Study the drawing (mm; zero at the part's minimum x, y, z) and answer. A direction names the side the tool comes from. Give positions to 0.01 mm unless a question says otherwise; leave off trailing zeros. Write each loop counter-clockwise with the first axis right and the second up, starting at its lowest first coordinate (ties: lowest second). Pieces come first, ordered by that corner, then holes.
1) Given pin 1 Ø1.5 at (y, z) = (9, 5) entering from -X; pin 2 Ø12 at (x, z) = (3, 5.5) entering from +Y; pin 3 Ø2 at (x, y) = (4.5, 14.5) entering from +Z, each flat-ended and moving along its own axis, determine where each tip first touches the part or whether it passes through.
2) Find section C-C (z = 16.5). Determine the outline of the cut face in (x, y).
3) Find section D-D (z = 6.5). Determine the outline of the cut face in (x, y).
4) A tool of negligible diameter and unlimited length cuts with its end or side. For the marked faces 1 and 2, from which of +Z, -Z, +X, -X, +Y, -Y can it reach the whole face along a straight path? Write none if from no direction.
5) Find section A-A (x = 12.5). Determine the outline of the cut face in (y, z).
6) Straight lines are drawn through the part: probe 1 along Z at (x, y) = (22.5, 14); probe 2 along X at (y, z) = (12.25, 5); probe 3 along Y at (x, z) = (14, 1.75). For each, find the intervals that lie inside material, in ascending order.
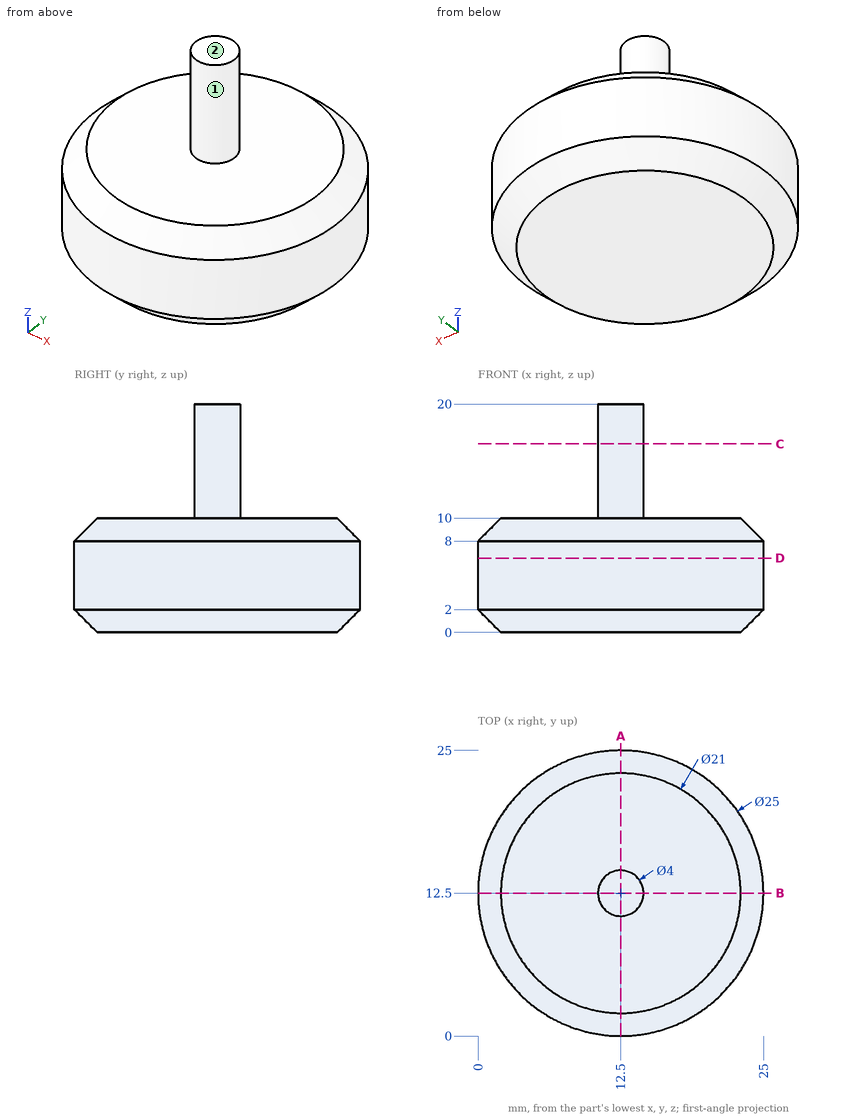
Results:
1. pin 1: stops at x = 0.31
1. pin 2: stops at y = 24.5
1. pin 3: stops at z = 10
2. outline: circle Ø4 at (12.5, 12.5)
3. outline: circle Ø25 at (12.5, 12.5)
4. face 1: +Z
4. face 2: +Z, +X, -X, +Y, -Y
5. outline: (0, 2) - (2, 0) - (23, 0) - (25, 2) - (25, 8) - (23, 10) - (14.5, 10) - (14.5, 20) - (10.5, 20) - (10.5, 10) - (2, 10) - (0, 8) - close
6. probe 1: z = 0 to 10
6. probe 2: x = 0 to 25
6. probe 3: y = 0.34 to 24.66
